Design review of the part built by this model. Coordinates are the model's own, in mm. A direction names the side the tool comes from. Coordinates: 2 decimals unless noted, no trailing zeros. Write each loop counter-clockwise with the first axis right and the second up, starting at its lowest first coordinate (ties: lowest second). Pieces come first, ordered by that corner, then holes.
Q1. Take a section at D-D (z = 165). Give the boundary of the cut face in (x, y).
Q2. Machinability: for faces 1 (the flat face through (30, -78, 170)), 2 (the flat face through (30, -71, 155)), 3 (the flat face through (30, 20, 2)), 4 (the flat face through (2, -43.01, 50)), 5 (the flat face through (23, -3, 155)), which of the approach directions +Z, -Z, +X, -X, +Y, -Y give a long, thin tool a straight path to every point of the face, cutting with its end or side? Answer none if there is none.
Q3. Take a section at B-B (y = -30). State how many separate pieces and enclosed holes the cut face has, and give its area (3 significant figures).
Q4. Take a section at C-C (x = -6). Give the boundary of the cut face in (y, z), and give its area (3 significant figures).
Q5. Take a section at A-A (z = 70). Give the boundary of the cut face in (x, y), and give its area (3 significant figures).
Q6. For probe 1 along Z at (x, y) = (51.5, -49.5); probe 2 along X at (y, z) = (-31, 48); probe 3 along Y at (x, z) = (-0.5, 79.5), list the stretches that pass through material, from the lowest coordinate up.
Q7. Mouldability with a two-part tool opening along Y and no side actions: class faces 6 (the flat face through (60, -31, 71)), 7 (the flat face through (30, -25, 170)), 8 (the flat face through (2, -30, 5)) as pulls with the +Y half, pulls with the -Y half, needs draft (parallel to the pull), parting line crosses it, or undercut.
Q8. Insertion check: pin 1 (11.5 mm diameter, centred on x = -16.5, y = -20, fed in from +Z); pin 2 (12 mm diameter, centred on x = -2, z = 19, fed in from -Y); pin 3 (1 mm diameter, centred on x = 32.5, y = 39, fed in from +Z). Each pin has a flat end and moves straight along its axis. Give the tip position at first contact, or say it passes through.
Autodesk Fusion 360 part; units mm, degrees
sketch "Sketch1" plane through (0, 0, 0) normal (0, 0, 1) x (1, 0, 0)
  line L0 (0, 0) -> (60, 0)
  line L1 (60, 0) -> (60, -60)
  line L2 (60, -60) -> (0, -60)
  line L3 (0, -60) -> (0, 0)
  dimension "d1" = 60
  dimension "d2" = 60
extrude "Extrude1" add sketch "Sketch1" along normal blind 155
sketch "Sketch2" plane through (0, 0, 0) normal (0, 0, 1) x (1, 0, 0)
  line L0 (0, 0) -> (30, 0)
  line L1 (30, 0) -> (30, -30)
  circle A0 centre (30, -30) radius 27.5
  dimension "d5" = 30
  dimension "d6" = 30
  dimension "d7" = 55
extrude "Extrude2" cut sketch "Sketch2" along normal through all
sketch "Sketch3" plane through (0, 0, 0) normal (1, 0, 0) x (0, 1, 0)
  line L0 (0, 0) -> (0, 5)
  line L1 (0, 5) -> (-10, 5)
  line L2 (-10, 5) -> (-50, 5)
  line L3 (-50, 5) -> (-50, 10)
  line L4 (-50, 10) -> (-10, 10)
  line L5 (-10, 10) -> (-10, 5)
  dimension "d9" = 10
  dimension "d10" = 5
  dimension "d11" = 40
  dimension "d12" = 5
extrude "Extrude3" cut sketch "Sketch3" along normal through all
sketch "Sketch4" plane through (0, 0, 0) normal (-1, 0, 0) x (0, -1, 0)
  line L0 (50, 10) -> (50, 5)
  line L1 (50, 5) -> (10, 5)
  line L2 (10, 5) -> (10, 10)
  line L3 (10, 10) -> (50, 10)
  line L4 (0, 0) -> (60, 0)
  line L5 (60, 0) -> (60, 155)
  line L6 (60, 155) -> (0, 155)
  line L7 (0, 155) -> (0, 0)
  line L8 (0.1, 82) -> (60, 82)
  line L9 (60, 82) -> (60, 12)
  line L10 (60, 12) -> (0.1, 12)
  line L11 (0.1, 12) -> (0.1, 82)
  line L12 (0.1, 82) -> (0, 155)
  line L13 (0.1, 82) -> (0, 82)
  dimension "d15" = 59.9
  dimension "d16" = 70
  dimension "d98" = 73
  dimension "d99" = 0.1
extrude "Extrude4" add sketch "Sketch4" along normal blind 27 contours L5 L8 L9 L10 L11
sketch "Sketch5" plane through (0, 0, 155) normal (0, 0, 1) x (-1, 0, 0)
  circle A0 centre (-30, 30) radius 27.5
  line L0 (0, 60) -> (-60, 60)
  line L1 (-60, 60) -> (-60, 0)
  line L2 (-60, 0) -> (0, 0)
  line L3 (0, 0) -> (0, 60)
  line L4 (27, 0.01) -> (25, 0.01)
  line L5 (25, 0.01) -> (25, 2.01)
  line L6 (25, 2.01) -> (2, 2.01)
  line L7 (2, 2.01) -> (2, 58.01)
  line L8 (2, 58.01) -> (25, 58.01)
  line L9 (25, 58.01) -> (25, 2.01)
  dimension "d19" = 2
  dimension "d20" = 2
  dimension "d21" = 23
  dimension "d22" = 56
extrude "Extrude5" cut sketch "Sketch5" against normal blind 138 contours L6 L7 L8 L9
sketch "Sketch6" plane through (0, -60, 0) normal (0, -1, 0) x (1, 0, 0)
  line L0 (0, 0) -> (60, 0)
  line L1 (60, 0) -> (60, 155)
  line L2 (60, 155) -> (0, 155)
  line L3 (0, 155) -> (0, 82)
  line L4 (0, 82) -> (-27, 82)
  line L5 (-27, 82) -> (-27, 12)
  line L6 (-27, 12) -> (0, 12)
  line L7 (0, 12) -> (0, 0)
sketch "Sketch7" plane through (60, 0, 0) normal (1, 0, 0) x (0, 1, 0)
  line L0 (-50, 5) -> (-50, 10)
  line L1 (-50, 10) -> (-10, 10)
  line L2 (-10, 10) -> (-10, 5)
  line L3 (-10, 5) -> (-50, 5)
  line L4 (-60, 0) -> (0, 0)
  line L5 (0, 0) -> (0, 155)
  line L6 (0, 155) -> (-60, 155)
  line L7 (-60, 155) -> (-60, 0)
sketch "Sketch8" plane through (0, -60, 0) normal (0, -1, 0) x (1, 0, 0)
sketch "Sketch9" plane through (0, -60, 0) normal (0, -1, 0) x (1, 0, 0)
sketch "Sketch10" plane through (0, 0, 0) normal (0, 1, 0) x (-1, 0, 0)
  line L0 (-60, 0) -> (0, 0)
  line L1 (0, 0) -> (0, 155)
  line L2 (0, 155) -> (-60, 155)
  line L3 (-60, 155) -> (-60, 0)
  line L4 (-10.5, 32) -> (-49.5, 32)
  line L5 (-49.5, 32) -> (-49.5, 0)
  line L6 (-49.5, 0) -> (-10.5, 0)
  line L7 (-10.5, 0) -> (-10.5, 32)
  line L8 (-10.5, 32) -> (-10.5, 155)
  line L9 (-10.5, 155) -> (0, 155)
  dimension "d26" = 39
  dimension "d27" = 32
  dimension "d100" = 10.5
  dimension "d101" = 123
extrude "Extrude6" add sketch "Sketch10" along normal blind 40 contours L0 L4 L5 L6 L7
sketch "Sketch11" plane through (0, 0, 155) normal (0, 0, 1) x (-1, 0, 0)
  line L0 (27, 60) -> (0, 60)
  line L1 (0, 60) -> (0, 0.1)
  line L2 (2, 2.01) -> (2, 58.01)
  line L3 (2, 58.01) -> (25, 58.01)
  line L4 (25, 58.01) -> (25, 2.01)
  line L5 (25, 2.01) -> (2, 2.01)
  line L6 (0, 0.1) -> (27, 0.1)
  line L7 (27, 0.1) -> (27, 60)
sketch "Sketch12" plane through (0, 0, 155) normal (0, 0, 1) x (-1, 0, 0)
sketch "Sketch13" plane through (0, 0, 155) normal (0, 0, 1) x (-1, 0, 0)
sketch "Sketch15" plane through (0, 0, 155) normal (0, 0, 1) x (-1, 0, 0)
  line L0 (-49.5, 0) -> (-47.5, 0)
  line L1 (-47.5, 0) -> (-47.5, -2)
  line L2 (-60, 0) -> (-49.5, 0)
  line L3 (-49.5, 0) -> (-49.5, -40)
  line L4 (-47.5, -2) -> (-12.5, -2)
  line L5 (-12.5, -2) -> (-12.5, -38)
  line L6 (-12.5, -38) -> (-47.5, -38)
  line L7 (-47.5, -38) -> (-47.5, -2)
  dimension "d34" = 2
  dimension "d35" = 2
  dimension "d36" = 35
  dimension "d37" = 36
extrude "Extrude7" cut sketch "Sketch15" against normal blind 153
sketch "Sketch16" plane through (0, 40, 0) normal (0, 1, 0) x (-1, 0, 0)
  line L0 (-10.5, 0) -> (-10.5, 32)
  line L1 (-10.5, 32) -> (-49.5, 32)
  line L2 (-49.5, 32) -> (-49.5, 0)
  line L3 (-49.5, 0) -> (-10.5, 0)
  line L4 (-49.5, 32) -> (-42, 32)
  line L5 (-42, 32) -> (-42, 28)
  line L6 (-42, 28) -> (-18, 28)
  line L7 (-18, 28) -> (-18, 4)
  line L8 (-18, 4) -> (-42, 4)
  line L9 (-42, 4) -> (-42, 28)
  dimension "d40" = 7.5
  dimension "d41" = 4
  dimension "d42" = 24
  dimension "d43" = 24
extrude "Extrude8" cut sketch "Sketch16" against normal blind 15 contours L6 L7 L8 L9
sketch "Sketch17" plane through (0, 2, 0) normal (0, 1, 0) x (-1, 0, 0)
  line L0 (-12.5, 32) -> (-47.5, 32)
  line L1 (-47.5, 32) -> (-47.5, 2)
  line L2 (-47.5, 2) -> (-12.5, 2)
  line L3 (-12.5, 2) -> (-12.5, 32)
  line L4 (-47.5, 32) -> (-28, 32)
  line L5 (-28, 32) -> (-28, 16)
  circle A0 centre (-28, 16) radius 5
  dimension "d46" = 19.5
  dimension "d47" = 16
  dimension "d48" = 10
extrude "Extrude9" cut sketch "Sketch17" against normal blind 12 contours A0
sketch "Sketch18" plane through (0, -60, 0) normal (0, -1, 0) x (1, 0, 0)
sketch "Sketch19" plane through (0, -60, 0) normal (0, -1, 0) x (1, 0, 0)
sketch "Sketch20" plane through (0, -60, 0) normal (0, -1, 0) x (1, 0, 0)
  line L0 (45.5, 51) -> (14.5, 51)
  line L1 (14.5, 51) -> (14.5, 0)
  line L2 (14.5, 0) -> (45.5, 0)
  line L3 (45.5, 0) -> (45.5, 51)
  line L4 (60, 0) -> (60, 155)
  line L5 (45.5, 51) -> (60, 51)
  line L6 (60, 51) -> (60, 155)
  dimension "d52" = 31
  dimension "d53" = 51
  dimension "d96" = 104
  dimension "d97" = 14.5
extrude "Extrude10" add sketch "Sketch20" along normal blind 22
sketch "Sketch21" plane through (0, 0, 155) normal (0, 0, 1) x (-1, 0, 0)
  line L0 (27, 60) -> (0, 60)
  line L1 (0, 60) -> (0, 0.1)
  line L2 (-14.5, 82) -> (-14.5, 80)
  line L3 (-14.5, 80) -> (-16.5, 80)
  line L4 (2, 2.01) -> (2, 58.01)
  line L5 (2, 58.01) -> (25, 58.01)
  line L6 (25, 58.01) -> (25, 2.01)
  line L7 (25, 2.01) -> (2, 2.01)
  line L8 (0, 0.1) -> (27, 0.1)
  line L9 (27, 0.1) -> (27, 60)
  line L10 (-12.5, -2) -> (-12.5, -38)
  line L11 (-12.5, -38) -> (-47.5, -38)
  line L12 (-47.5, -38) -> (-47.5, -2)
  line L13 (-47.5, -2) -> (-12.5, -2)
  line L14 (-10.5, 0) -> (-49.5, 0)
  line L15 (-49.5, 0) -> (-49.5, -40)
  line L16 (-49.5, -40) -> (-10.5, -40)
  line L17 (-10.5, -40) -> (-10.5, 0)
  dimension "d56" = 2
  dimension "d57" = 2
sketch "Sketch22" plane through (0, 0, 155) normal (0, 0, 1) x (-1, 0, 0)
  line L0 (-16.5, 80) -> (-43.5, 80)
  line L1 (-43.5, 80) -> (-43.5, 62)
  line L2 (-43.5, 62) -> (-16.5, 62)
  line L3 (-16.5, 62) -> (-16.5, 80)
  dimension "d58" = 27
  dimension "d59" = 18
extrude "Extrude11" cut sketch "Sketch22" against normal blind 153
sketch "Sketch24" plane through (0, 0, 155) normal (0, 0, 1) x (1, 0, 0)
sketch "Sketch26" plane through (-2, 0, 0) normal (-1, 0, 0) x (0, -1, 0)
  line L0 (58.01, 82) -> (2.01, 82)
  line L1 (2.01, 82) -> (2.01, 17)
  line L2 (2.01, 17) -> (58.01, 17)
  line L3 (58.01, 17) -> (58.01, 82)
  line L4 (2.01, 155) -> (2.01, 80)
  line L5 (2.01, 80) -> (7.01, 80)
  line L6 (7.01, 80) -> (17.01, 80)
  line L7 (17.01, 80) -> (17.01, 20)
  line L8 (17.01, 20) -> (7.01, 20)
  line L9 (7.01, 20) -> (7.01, 80)
  line L10 (30.01, 155) -> (30.01, 17)
  line L11 (2.01, 155) -> (58.01, 155)
  line L12 (43.01, 80) -> (43.01, 20)
  line L13 (53.01, 80) -> (43.01, 80)
  line L14 (53.01, 20) -> (53.01, 80)
  line L15 (43.01, 20) -> (53.01, 20)
  dimension "d66" = 75
  dimension "d67" = 5
  dimension "d68" = 10
  dimension "d69" = 60
extrude "Extrude14" cut sketch "Sketch26" against normal blind 25 contours L12 L13 L14 L15
extrude "Extrude13" cut sketch "Sketch26" against normal blind 25 contours L6 L7 L8 L9
sketch "Sketch27" plane through (60, 0, 0) normal (1, 0, 0) x (0, 1, 0)
  line L0 (-60, 155) -> (-50, 155)
  line L1 (-50, 155) -> (-10, 155)
  line L2 (-10, 155) -> (-10, 110)
  line L3 (-10, 110) -> (-50, 110)
  line L4 (-50, 110) -> (-50, 155)
  dimension "d74" = 10
  dimension "d75" = 40
  dimension "d76" = 45
extrude "Extrude15" cut sketch "Sketch27" against normal blind 20
sketch "Sketch28" plane through (0, 0, 155) normal (0, 0, 1) x (-1, 0, 0)
  line L0 (-60, 30) -> (0, 30) construction
  line L1 (-60, 60) -> (-60, 0)
  line L2 (0, 30) -> (0, 25)
  line L3 (0, 25) -> (-60, 25)
  line L4 (-60, 25) -> (-60, 81)
  line L5 (-60, 81) -> (0, 81)
  line L6 (0, 81) -> (0, 25)
  dimension "d79" = 5
  dimension "d80" = 60
  dimension "d81" = 56
extrude "Extrude16" add sketch "Sketch28" along normal blind 30
sketch "Sketch29" plane through (0, 0, 155) normal (0, 0, 1) x (-1, 0, 0)
sketch "Sketch30" plane through (0, 0, 0) normal (-1, 0, 0) x (0, -1, 0)
  line L0 (60, 82) -> (60, 155)
  line L1 (60, 12) -> (0.1, 12)
  line L2 (0.1, 12) -> (0.1, 82)
  line L3 (0.1, 82) -> (60, 82)
  line L4 (0, 155) -> (0, 0)
  line L5 (0, 0) -> (60, 0)
  line L6 (60, 155) -> (81, 155)
  line L7 (81, 155) -> (81, 185)
  line L8 (81, 185) -> (25, 185)
  line L9 (25, 185) -> (25, 155)
  line L10 (50, 10) -> (50, 5)
  line L11 (50, 5) -> (10, 5)
  line L12 (10, 5) -> (10, 10)
  line L13 (10, 10) -> (50, 10)
  line L14 (25, 185) -> (28, 185)
  line L15 (28, 185) -> (28, 182)
  line L16 (28, 182) -> (78, 182)
  line L17 (78, 182) -> (78, 158)
  line L18 (78, 158) -> (28, 158)
  line L19 (28, 158) -> (28, 182)
  line L20 (25, 155) -> (0, 155)
  line L21 (60, 0) -> (60, 12)
  dimension "d84" = 3
  dimension "d85" = 3
  dimension "d86" = 50
  dimension "d87" = 24
extrude "Extrude17" cut sketch "Sketch30" against normal through all contours L16 L17 L18 L19
sketch "Sketch31" plane through (60, 0, 0) normal (1, 0, 0) x (0, 1, 0)
sketch "Sketch32" plane through (0, 0, 185) normal (0, 0, 1) x (-1, 0, 0)
  line L0 (0, 81) -> (-60, 81)
  line L1 (-60, 81) -> (-60, 25)
  line L2 (-60, 25) -> (0, 25)
  line L3 (0, 25) -> (0, 81)
  line L4 (0, 25) -> (-60, 25)
  line L5 (-60, 25) -> (-60, 48)
  line L6 (-60, 48) -> (0, 48)
  line L7 (0, 48) -> (0, 25)
  dimension "d89" = 60
  dimension "d90" = 23
sketch "Sketch33" plane through (0, 0, 158) normal (0, 0, 1) x (-1, 0, 0)
  line L0 (-60, 78) -> (-60, 28)
  line L1 (-60, 28) -> (0, 28)
  line L2 (0, 28) -> (0, 78)
  line L3 (0, 78) -> (-60, 78)
  line L4 (0, 28) -> (-5, 28)
  line L5 (-5, 28) -> (-53, 28)
  line L6 (-53, 28) -> (-53, 40)
  line L7 (-53, 40) -> (-5, 40)
  line L8 (-5, 40) -> (-5, 28)
  dimension "d93" = 48
  dimension "d94" = 12
extrude "Extrude19" cut sketch "Sketch33" against normal through all contours L1 L5 L6 L7 L8
equation "d23 = -65.00 mm - 73 mm"
equation "d38 = -30.00 mm - 123 mm"
equation "d60 = -49.00 mm - 50 mm - 54 mm"
Response:
1. outline: (0, -81) - (60, -81) - (60, -78) - (0, -78) - close; (0, -28) - (60, -28) - (60, -25) - (0, -25) - close
2. face 1: +X, -X
2. face 2: +X, -X, -Y
2. face 3: +Z
2. face 4: none
2. face 5: +Z, +X, -X, +Y
3. separate pieces: 6
3. enclosed holes: 0
3. area: 1,250 mm2
4. outline: (-60, 12) - (-0.1, 12) - (-0.1, 82) - (-2.01, 82) - (-2.01, 17) - (-58.01, 17) - (-58.01, 82) - (-60, 82) - close
4. area: 553 mm2
5. outline: (-27, -60) - (60, -60) - (60, 0) - (0, 0) - (0, -0.1) - (-27, -0.1) - close; (-2, -43.01) - (5.77, -43.01) arc R27.5 cw to (5.76, -17.01) - (-2, -17.01) - close; hole (-25, -58.01) - (-2, -58.01) - (-2, -53.01) - (14.94, -53.01) arc R27.5 ccw (long way) to (14.91, -7.01) - (-2, -7.01) - (-2, -2.01) - (-25, -2.01) - close
5. area: 1,320 mm2
6. probe 1: z = 0 to 5, 10 to 110, 155 to 158, 182 to 185
6. probe 2: x = -27 to -25, -2 to 2.52, 57.48 to 60
6. probe 3: y = -60 to -53.01, -43.01 to -17.01, -7.01 to -0.1
7. face 6: needs draft
7. face 7: pulls with the +Y half
7. face 8: undercut
8. pin 1: stops at z = 17
8. pin 2: stops at y = -60
8. pin 3: stops at z = 32
